Work out the finished part from the listing and answer in its coordinate system (mm). A direction names the side the tool comes from. Coordinates: 2 decimals unless noted, no trailing zeros. Order: outer loops, then holes, each group sorted by start corner. A loop starts at its lowest first (then second) coordinate and runs counter-clockwise, first axis right, second up. Notation, with made-up numbers: (9.25, 30) -> (16.25, 30) arc R20 cw to (16.25, 68) -> close; hole circle Ø3 at (-19, 76.25). An arc over 180 degrees is marked (long way). Use one line per item in the form item = value.
from build123d import *

# Parameters (mm, degrees)
BOSS_EXTRUDE1_DEPTH = 1.2


with BuildPart() as part:
    # Sketch1 → Boss-Extrude1 (new body)
    with BuildSketch(Plane(origin=(0, 0, 0), x_dir=(1, 0, 0), z_dir=(0, 1, 0))):
        with BuildLine():
            Line((-0.75, 2.54), (-7.25, 2.54))
            ThreePointArc((-7.25, 2.54), (-7.780330086, 2.759669914), (-8, 3.29))
            Line((-8, 3.29), (-8, 4.33))
            ThreePointArc((-8, 4.33), (-7.780330086, 4.860330086), (-7.25, 5.08))
            Line((-7.25, 5.08), (-0.75, 5.08))
            ThreePointArc((-0.75, 5.08), (-0.219669914, 5.299669914), (0, 5.83))
            Line((0, 5.83), (0, 7.62000013))
            ThreePointArc((0, 7.62000013), (-0.219669914, 8.150330216), (-0.75, 8.37000013))
            Line((-0.75, 8.37000013), (-7.25, 8.37000013))
            ThreePointArc((-7.25, 8.37000013), (-7.780330086, 8.589670044), (-8, 9.12000013))
            Line((-8, 9.12000013), (-8, 10.16000013))
            ThreePointArc((-8, 10.16000013), (-7.780330086, 10.690330216), (-7.25, 10.91000013))
            Line((-7.25, 10.91000013), (-0.75, 10.91000013))
            ThreePointArc((-0.75, 10.91000013), (-0.219669868, 11.12967009), (0, 11.66000026))
            Line((0, 11.66000026), (0, 13.45000026))
            ThreePointArc((0, 13.45000026), (-0.219669914, 13.980330346), (-0.75, 14.20000026))
            Line((-0.75, 14.20000026), (-7.25, 14.20000026))
            ThreePointArc((-7.25, 14.20000026), (-7.780330086, 14.419670174), (-8, 14.95000026))
            Line((-8, 14.95000026), (-8, 15.99000026))
            ThreePointArc((-8, 15.99000026), (-7.780330086, 16.520330346), (-7.25, 16.74000026))
            Line((-7.25, 16.74000026), (-0.75, 16.74000026))
            ThreePointArc((-0.75, 16.74000026), (-0.219669868, 16.95967022), (0, 17.49000039))
            Line((0, 17.49000039), (0, 19.28000039))
            ThreePointArc((0, 19.28000039), (-0.219669914, 19.810330476), (-0.75, 20.03000039))
            Line((-0.75, 20.03000039), (-7.25, 20.03000039))
            ThreePointArc((-7.25, 20.03000039), (-7.780330086, 20.249670304), (-8, 20.78000039))
            Line((-8, 20.78000039), (-8, 21.82000039))
            ThreePointArc((-8, 21.82000039), (-7.780330086, 22.350330476), (-7.25, 22.57000039))
            Line((-7.25, 22.57000039), (-0.75, 22.57000039))
            ThreePointArc((-0.75, 22.57000039), (-0.219669868, 22.78967035), (0, 23.32000052))
            Line((0, 23.32000052), (0, 25.11000052))
            ThreePointArc((0, 25.11000052), (-0.219669914, 25.640330606), (-0.75, 25.86000052))
            Line((-0.75, 25.86000052), (-7.25, 25.86000052))
            ThreePointArc((-7.25, 25.86000052), (-7.780330086, 26.079670434), (-8, 26.61000052))
            Line((-8, 26.61000052), (-8, 27.65000052))
            ThreePointArc((-8, 27.65000052), (-7.780330086, 28.180330606), (-7.25, 28.40000052))
            Line((-7.25, 28.40000052), (-0.75, 28.40000052))
            ThreePointArc((-0.75, 28.40000052), (-0.219669868, 28.61967048), (0, 29.15000065))
            Line((0, 29.15000065), (0, 30.94000065))
            ThreePointArc((0, 30.94000065), (-0.219669914, 31.470330736), (-0.75, 31.69000065))
            Line((-0.75, 31.69000065), (-7.25, 31.69000065))
            ThreePointArc((-7.25, 31.69000065), (-7.780330086, 31.909670564), (-8, 32.44000065))
            Line((-8, 32.44000065), (-8, 33.48000065))
            ThreePointArc((-8, 33.48000065), (-7.780330086, 34.010330736), (-7.25, 34.23000065))
            Line((-7.25, 34.23000065), (-0.75, 34.23000065))
            ThreePointArc((-0.75, 34.23000065), (-0.219669868, 34.44967061), (0, 34.98000078))
            Line((0, 34.98000078), (0, 36.77000078))
            ThreePointArc((0, 36.77000078), (-0.219669914, 37.300330866), (-0.75, 37.52000078))
            Line((-0.75, 37.52000078), (-7.25, 37.52000078))
            ThreePointArc((-7.25, 37.52000078), (-7.780330086, 37.739670694), (-8, 38.27000078))
            Line((-8, 38.27000078), (-8, 39.31000078))
            ThreePointArc((-8, 39.31000078), (-7.780330086, 39.840330866), (-7.25, 40.06000078))
            Line((-7.25, 40.06000078), (-0.75, 40.06000078))
            ThreePointArc((-0.75, 40.06000078), (-0.219669868, 40.27967074), (0, 40.81000091))
            Line((0, 40.81000091), (0, 42.60000091))
            ThreePointArc((0, 42.60000091), (-0.219669914, 43.130330995), (-0.75, 43.35000091))
            Line((-0.75, 43.35000091), (-7.25, 43.35000091))
            ThreePointArc((-7.25, 43.35000091), (-7.780330086, 43.569670824), (-8, 44.10000091))
            Line((-8, 44.10000091), (-8, 45.14000091))
            ThreePointArc((-8, 45.14000091), (-7.780330086, 45.670330995), (-7.25, 45.89000091))
            Line((-7.25, 45.89000091), (-0.75, 45.89000091))
            ThreePointArc((-0.75, 45.89000091), (-0.219669868, 46.10967087), (0, 46.64000104))
            Line((0, 46.64000104), (0, 48.43000104))
            ThreePointArc((0, 48.43000104), (-0.219669914, 48.960331125), (-0.75, 49.18000104))
            Line((-0.75, 49.18000104), (-7.25, 49.18000104))
            ThreePointArc((-7.25, 49.18000104), (-7.780330086, 49.399670954), (-8, 49.93000104))
            Line((-8, 49.93000104), (-8, 50.97000104))
            ThreePointArc((-8, 50.97000104), (-7.780330086, 51.500331125), (-7.25, 51.72000104))
            Line((-7.25, 51.72000104), (-0.75, 51.72000104))
            ThreePointArc((-0.75, 51.72000104), (-0.219669868, 51.939671), (0, 52.470001169))
            Line((0, 52.470001169), (0, 54.260001169))
            ThreePointArc((0, 54.260001169), (-0.219669914, 54.790331255), (-0.75, 55.010001169))
            Line((-0.75, 55.010001169), (-7.25, 55.010001169))
            ThreePointArc((-7.25, 55.010001169), (-7.780330086, 55.229671084), (-8, 55.760001169))
            Line((-8, 55.760001169), (-8, 56.800001169))
            ThreePointArc((-8, 56.800001169), (-7.780330086, 57.330331255), (-7.25, 57.550001169))
            Line((-7.25, 57.550001169), (-0.75, 57.550001169))
            ThreePointArc((-0.75, 57.550001169), (-0.219669914, 57.769671084), (0, 58.300001169))
            Line((0, 58.300001169), (0, 60.090001169))
            ThreePointArc((0, 60.090001169), (0.219669914, 60.620331255), (0.75, 60.840001169))
            Line((0.75, 60.840001169), (14.25, 60.840001169))
            ThreePointArc((14.25, 60.840001169), (14.780330086, 60.620331255), (15, 60.090001169))
            Line((15, 60.090001169), (15, 0))
            Line((15, 0), (15, -7.25))
            ThreePointArc((15, -7.25), (14.780330086, -7.780330086), (14.25, -8))
            Line((14.25, -8), (0.75, -8))
            ThreePointArc((0.75, -8), (0.219669914, -7.780330086), (0, -7.25))
            Line((0, -7.25), (0, 0))
            Line((0, 0), (0, 1.79))
            ThreePointArc((0, 1.79), (-0.219669914, 2.320330086), (-0.75, 2.54))
        make_face()
    extrude(amount=BOSS_EXTRUDE1_DEPTH)


solid = part.part
(1) Straight lines are drawn through the part: line 1 along X through (y, z) = (0.25, -42.5); line 2 along X through (y, z) = (0.1, -5); line 3 along Z through (x, y) = (0.25, 0.5). For each, find the intervals that lie inside material, in ascending order.
Data:
line_1 = 0 to 15
line_2 = -7.59 to 15
line_3 = -60.65 to 7.81
(2) Which of the six approach directions +Z, -Z, +X, -X, +Y, -Y give full straight-line access (tool end or side, diameter ignored) to faces 1 (the flat face through (-4, 1, -55.01)), 2 (the flat face through (-4, 1, -57.55)), 3 (the flat face through (8, 1, 8))?
Data:
face_1 = -X, +Y, -Y
face_2 = -Z, -X, +Y, -Y
face_3 = +Z, +X, -X, +Y, -Y
(3) The mould has two halves that part along Z. Classify faces 4 (the flat face through (-4, 1, -8.37)), 5 (the flat face through (0, 1, 3)), 6 (the flat face through (-4, 1, -2.54)), 7 (the flat face through (7, 1, -60.84)): released by +Z, released by -Z, zero draft, split by the parting line, or undercut.
Data:
face_4 = undercut
face_5 = zero draft
face_6 = released by +Z
face_7 = released by -Z
(4) Each of these flat-tipped pins is pushed along its axis until it touches: P1, Ø10, axis at x = 2, z = -45.5, coming from the -Y side; P2, Ø0.6, axis at x = -3.5, y = 0.5, coming from the +Z side; P3, Ø0.6, axis at x = -2.5, y = 0.5, coming from the -Z side; P4, Ø1.5, axis at x = -1.5, z = 1, coming from the -Y side. Where does it stop, or does it pass through?
Data:
P1 = 0
P2 = -2.54
P3 = -57.55
P4 = through
(5) Section B-B on z = -30 is taken. Write down the section's boundary in (x, y), plus the area to 3 significant figures.
Data:
outline = (0, 0) -> (15, 0) -> (15, 1.2) -> (0, 1.2) -> close
area = 18.0 mm²
(6) Section A-A on x = -2 is taken. Count the separate pieces of the cut face and the enclosed holes in it, plus the area to 3 significant figures.
Data:
separate_pieces = 10
enclosed_holes = 0
area = 30.5 mm²
